Design review of the part shown in the three views and the two pictorial views. Dimensions are in mm from the part's minimum x, y and z. A direction names the side the tool comes from. Give positions to 0.01 mm unless a question says otherwise; leave off trailing zeros. Loops run counter-clockwise (first coordinate to the right, second up) from the corner with the lowest first, then second, coordinate; pieces in that order, holes last. Notation, with made-up numbers: (-34.75, 16.25) -> (-14.75, 16.25) arc R4 ccw to (-14.75, 21.25) -> close; hole circle Ø4 at (-17, -24.5). An arc over 180 degrees is marked (long way). Answer as CSV lines item,"result". Start each with the question number.
Item 1: Add section D-D on z = 15. State the section outline as (x, y) points (3 decimals).
Item 2: Add section B-B on z = 21. State the section outline as (x, y) points (3 decimals), plus the area to 3 significant figures.
Item 3: Add section A-A on x = 26. State the section outline as (y, z) points (3 decimals), plus the area to 3 significant figures.
Item 4: For L1, parallel to Z at x = 19.05, y = 1.8 (3 decimals); L2, parallel to Z at x = 4, y = 10 (3 decimals), list the stretches that pass through material, from the lowest coordinate up. Write a range as from..to.
Item 5: Add section C-C on x = 19.05. State the section outline as (y, z) points (3 decimals).
Item 6: Clearance check with flat-ended pins moving along their axes: P1, Ø8, axis at x = 17.5, y = 8, coming from the +Z side (3 decimals); P2, Ø12, axis at x = 17.5, z = 22.5, coming from the +Y side (3 decimals). State where each tip first meets the part, or that it passes through.
Item 7: Machinability: for the marked faces 1 and 2, which of the approach directions +Z, -Z, +X, -X, +Y, -Y give a long, thin tool a straight path to every point of the face, cutting with its end or side? Answer none if there is none.
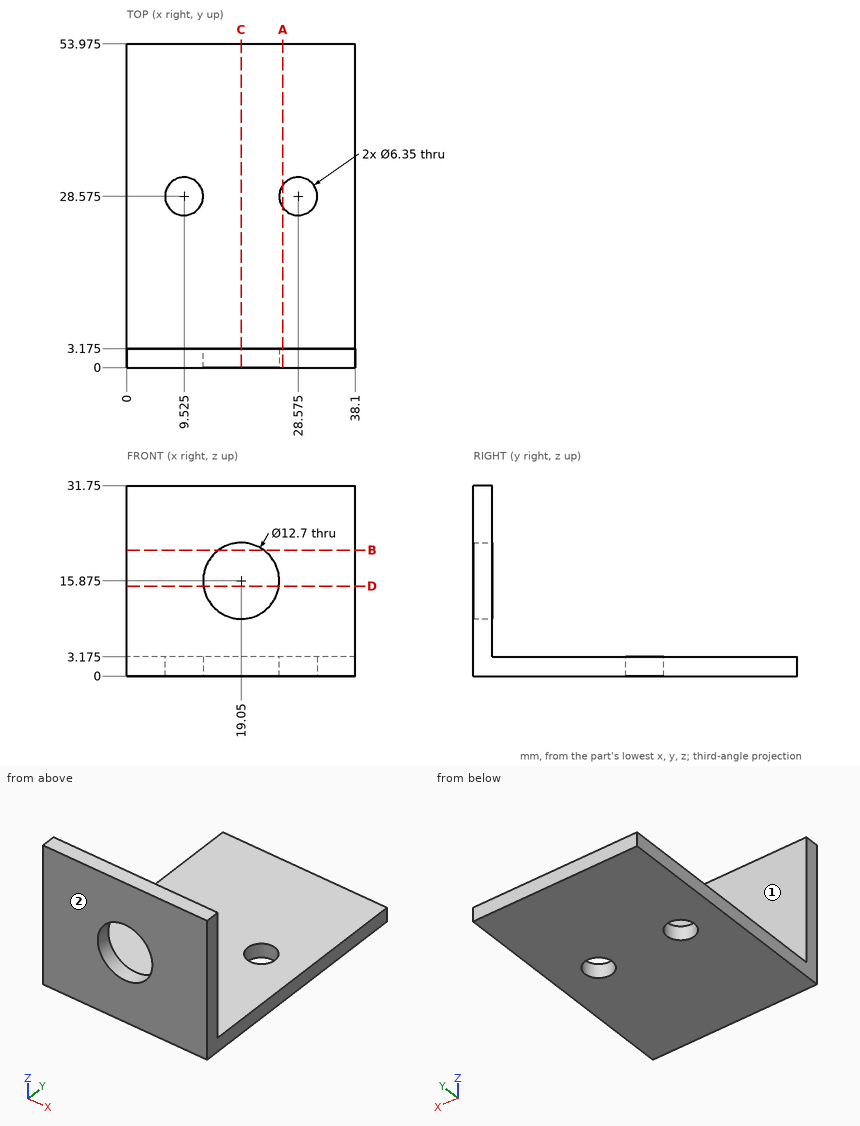
Computed values:
1,outline,"(0, 0) -> (12.761, 0) -> (12.761, 3.175) -> (0, 3.175) -> close; (25.339, 0) -> (38.1, 0) -> (38.1, 3.175) -> (25.339, 3.175) -> close"
2,outline,"(0, 0) -> (15.301, 0) -> (15.301, 3.175) -> (0, 3.175) -> close; (22.799, 0) -> (38.1, 0) -> (38.1, 3.175) -> (22.799, 3.175) -> close"
2,area,"97.2 mm²"
3,outline,"(0, 0) -> (26.718, 0) -> (26.718, 3.175) -> (3.175, 3.175) -> (3.175, 31.75) -> (0, 31.75) -> close; (30.432, 0) -> (53.975, 0) -> (53.975, 3.175) -> (30.432, 3.175) -> close"
3,area,"250 mm²"
4,L1,"0..9.525, 22.225..31.75"
4,L2,"0..3.175"
5,outline,"(0, 0) -> (53.975, 0) -> (53.975, 3.175) -> (3.175, 3.175) -> (3.175, 9.525) -> (0, 9.525) -> close; (0, 22.225) -> (3.175, 22.225) -> (3.175, 31.75) -> (0, 31.75) -> close"
6,P1,"z = 3.175"
6,P2,"y = 3.175"
7,face 1,"+Z, +X, -X, +Y"
7,face 2,"+Z, -Z, +X, -X, -Y"
